CAD build for the part. Positions are in the model's coordinates, mm. A direction names the side the tool comes from. Coordinates: 2 decimals unless noted, no trailing zeros. Loops run counter-clockwise (first coordinate to the right, second up) from the corner with the lowest first, then second, coordinate; pieces in that order, holes last. Notation, with made-up numbers: (-18.5, -36.5) - (-10.5, -36.5) arc R5 cw to (-10.5, -32.5) - close; hole circle Ø7 at (9.25, -13). An arc over 180 degrees is marked (long way). Put each result on its own line as item: value.
```python
from build123d import *

# Parameters (mm, degrees)
BOSS_EXTRUDE1_DEPTH = 32
SKETCH2_R           = 9.5
CUT_EXTRUDE1_DEPTH  = 64
CUT_EXTRUDE2_DEPTH  = 22
CUT_EXTRUDE3_START  = -50
CUT_EXTRUDE3_DEPTH  = 38
CHAMFER1_SIZE       = 2


with BuildPart() as part:
    # Sketch1 → Boss-Extrude1 (new, symmetric)
    with BuildSketch(Plane.XY):
        with BuildLine():
            Line((-36, 0), (-32, 0))
            ThreePointArc((-32, 0), (0, 32), (32, 0))
            Line((32, 0), (36, 0))
            Line((36, 0), (36, 32))
            Line((36, 32), (72, 32))
            Line((72, 32), (72, 52))
            Line((72, 52), (36, 52))
            ThreePointArc((36, 52), (0, 64.524731996), (-36, 52))
            Line((-36, 52), (-72, 52))
            Line((-72, 52), (-72, 32))
            Line((-72, 32), (-36, 32))
            Line((-36, 32), (-36, 0))
        make_face()
    extrude(amount=BOSS_EXTRUDE1_DEPTH, both=True)

    # Sketch2 → Cut-Extrude1 (cut)
    with BuildSketch(Plane(origin=(0, 52, 0), x_dir=(1, 0, 0), z_dir=(0, 1, 0))):
        with Locations(Location((-54, 0, 0), (0, 0, 270))):
            Circle(SKETCH2_R)
        with Locations(Location((54, 0, 0), (0, 0, 270))):
            Circle(SKETCH2_R)
    extrude(amount=-CUT_EXTRUDE1_DEPTH, mode=Mode.SUBTRACT)

    # Sketch3 → Cut-Extrude2 (cut)
    with BuildSketch(Plane(origin=(0, 52, 0), x_dir=(1, 0, 0), z_dir=(0, 1, 0))):
        with BuildLine():
            ThreePointArc((-72, -4.4e-08), (-70.099431041, 16.433799554), (-64.498061986, 32))
            Line((-64.498061986, 32), (-72, 32))
            Line((-72, 32), (-72, -4.4e-08))
        make_face()
        with BuildLine():
            Line((-72, -32), (-64.498061986, -32))
            ThreePointArc((-64.498061986, -32), (-70.099431031, -16.433799597), (-72, -4.4e-08))
            Line((-72, -4.4e-08), (-72, -32))
        make_face()
        with BuildLine():
            Line((72, 32), (64.498061986, 32))
            ThreePointArc((64.498061986, 32), (70.099431036, 16.433799576), (72, 0))
            Line((72, 0), (72, 32))
        make_face()
        with BuildLine():
            ThreePointArc((72, 0), (70.099431036, -16.433799576), (64.498061986, -32))
            Line((64.498061986, -32), (72, -32))
            Line((72, -32), (72, 0))
        make_face()
    extrude(amount=-CUT_EXTRUDE2_DEPTH, mode=Mode.SUBTRACT)

    # Sketch5 → Cut-Extrude3 (cut)
    with BuildSketch(Plane(origin=(0, 0, -32), x_dir=(-1, 0, 0), z_dir=(0, 0, -1)).offset(CUT_EXTRUDE3_START)):
        with BuildLine():
            Line((-34, 0), (-32, 0))
            ThreePointArc((-32, 0), (0, 32), (32, 0))
            Line((32, 0), (34, 0))
            ThreePointArc((34, 0), (0, 34), (-34, 0))
        make_face()
    extrude(amount=CUT_EXTRUDE3_DEPTH, mode=Mode.SUBTRACT)

    # Chamfer1
    chamfer1_edges = [part.edges().sort_by_distance(p)[0] for p in [
        (0, 32, 18),
        (0, 32, -20),
    ]]
    chamfer(chamfer1_edges, length=CHAMFER1_SIZE - 0.0001)  # a hair under: the kernel refuses the full size


solid = part.part
```
Q1. Slice it at A-A, the plane x = -54. Give the cut face in (y, z), then the cut area to 3 significant figures.
Determined:
outline: (32, -32) - (52, -32) - (52, -9.5) - (32, -9.5) - close; (32, 9.5) - (52, 9.5) - (52, 32) - (32, 32) - close
area: 900 mm2
Q2. Wall check: L1, parallel to X at y = 34.5, z = 5; L2, parallel to Y at x = -44, z = 5.5; L3, parallel to Z at x = -11.5, y = 31. Give the ranges that are in metal, low to high. Write a range as from..to.
Determined:
L1: -71.83..-62.08, -45.92..45.92, 62.08..71.83
L2: 32..52
L3: -32..-20.94, 18.94..32
Q3. Tool access for faces 1 (the flat face through (-46, 32, -7)), 2 (the flat face through (36, 16, 0)), 3 (the flat face through (46, 52, -7)), 4 (the conical face through (0.71, 32.31, -21.68)): list every direction of +Z, -Z, +X, -X, +Y, -Y with a clear straight run to the whole face (end or side of a thin tool).
Determined:
face 1: +Z, -Z, -X, -Y
face 2: +Z, -Z, +X, -Y
face 3: +Z, -Z, +X, +Y
face 4: -Y
Q4. Pin check, flat tips, straight feed: pin 1 Ø2 at (x, z) = (-24.5, -11.5) entering from -Y; pin 2 Ø10 at (y, z) = (11, -4) entering from -X; pin 3 Ø6 at (y, z) = (41.5, 7) entering from +X. Stop position of each tip, or through.
Determined:
pin 1: y = 22.49
pin 2: x = -36
pin 3: x = 71.89
Q5. Slice it at B-B, the plane y = 38. Give the cut face in (x, z).
Determined:
outline: (-64.5, -32) - (64.5, -32) arc R72 ccw to (64.5, 32) - (-64.5, 32) arc R72 ccw to start; hole circle Ø19 at (-54, 0); hole circle Ø19 at (54, 0)
Q6. Slice it at C-C, the plane z = -11.5. Give the cut face in (x, y).
Determined:
outline: (-71.08, 32) - (-36, 32) - (-36, 0) - (-34, 0) arc R34 cw to (34, 0) - (36, 0) - (36, 32) - (71.08, 32) - (71.08, 52) - (36, 52) arc R58 ccw to (-36, 52) - (-71.08, 52) - close
Q7. Mould opens along X. For faces 5 (the flat face through (46, 32, 8)), 6 (the cylindrical face through (0.544, 64.522, 0.448)), 7 (the cylindrical face through (-0.704, 31.992, -26.93)) say: +X half, -X half, draft (parallel to the pull), parting line (faces both ways), or undercut.
Determined:
face 5: draft
face 6: parting line
face 7: undercut
Q8. Slice it at D-D, the plane x = 46. Give the cut face in (y, z).
Determined:
outline: (32, -32) - (52, -32) - (52, -5.12) - (32, -5.12) - close; (32, 5.12) - (52, 5.12) - (52, 32) - (32, 32) - close
